Can you work these out from the drawing? Everything is in mm from the part's minimum corner. Coordinates: 2 decimals unless noted, no trailing zeros. Loops run counter-clockwise (first coordinate to the right, second up) from the corner with the lowest first, then second, coordinate; pieces in that order, holes last.
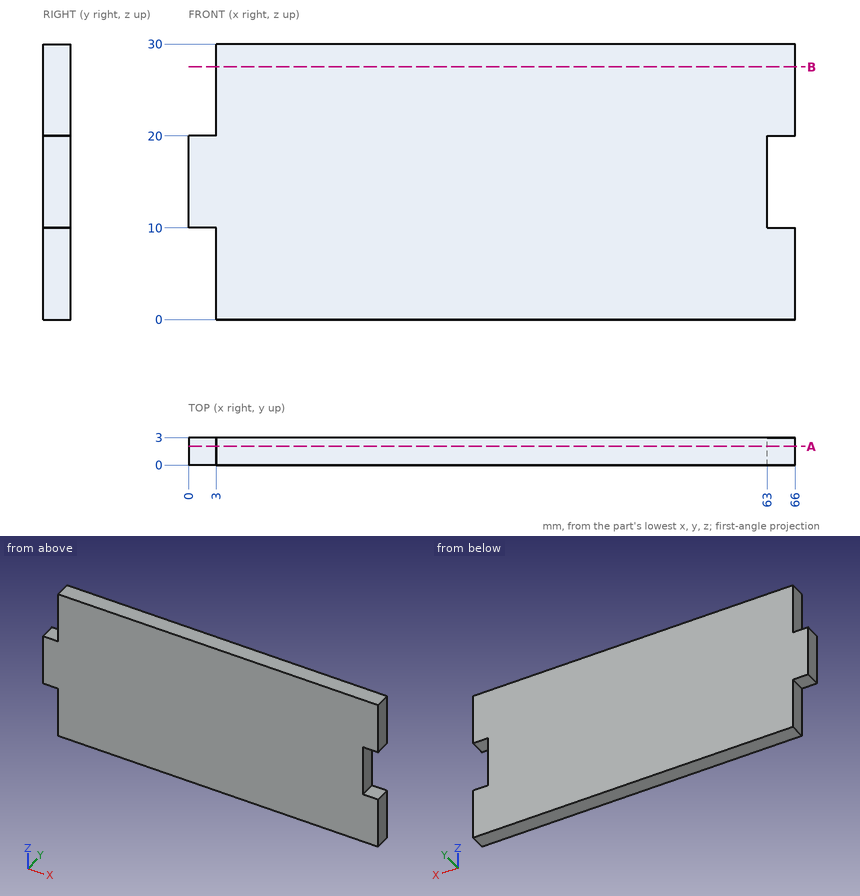
1. For pin 1 (1.5 mm diameter, centred on y = 2, z = 4, fed in from -X), with a flat end and sliding along its axis, tell me the tip position at first contact or that it passes through.
2. I want a section at B-B (z = 27.5). Please give me the cut outline in (x, y), then the cut area to 3 significant figures.
3. I need wall thicknesses on line 1 along Z through (x, y) = (63.5, 1); line 2 along X through (y, z) = (0.55, 15.5); line 3 along X through (y, z) = (0.35, 6.25). Which ranges of each line are inside material? Lowest first, please.
4. I want a section at A-A (y = 2.05). Please give me the cut outline in (x, z), then the cut area to 3 significant figures.
Response values:
1. pin 1: stops at x = 3
2. outline: (3, 0) - (66, 0) - (66, 3) - (3, 3) - close
2. area: 189 mm2
3. line 1: z = 0 to 10, 20 to 30
3. line 2: x = 0 to 63
3. line 3: x = 3 to 66
4. outline: (0, 10) - (3, 10) - (3, 0) - (66, 0) - (66, 10) - (63, 10) - (63, 20) - (66, 20) - (66, 30) - (3, 30) - (3, 20) - (0, 20) - close
4. area: 1,890 mm2
